CAD build for the part. Positions are in the model's coordinates, mm. Face numbers are marked on the shaded views. A direction names the side the tool comes from. Coordinates: 2 decimals unless noted, no trailing zeros. Write each loop counter-clockwise with the first axis right and the second up, starting at its lowest first coordinate (ties: lowest second). Pieces come first, ordered by that corner, then holes. Notation, with made-up numbers: (46.25, 82.5) -> (51.25, 82.5) arc R26 cw to (51.25, 113.5) -> close; hole circle Ø10 at (81.25, -1). An arc over 180 degrees is marked (long way). Answer as CSV lines item,"result".
```python
from build123d import *

# Parameters (mm, degrees)
EXTRUSION1_DEPTH = 35
ESQUISSE2_R      = 2
EXTRUSION2_DEPTH = 17
ESQUISSE4_R      = 1.5
ESQUISSE4_R_2    = 2.5
ESQUISSE4_W      = 17.5
ESQUISSE4_H      = 20
EXTRUSION3_DEPTH = 17


with BuildPart() as part:
    # Esquisse1 → Extrusion1 (new body)
    with BuildSketch(Plane.XY):
        Polygon((-13.454581117, 9.773157895), (-13.454581117, -10.226842105), (5.545418883, -10.226842105), (5.545418883, -8.726842105), (-11.954581117, -8.726842105), (-11.954581117, 9.773157895), align=None)
    extrude(amount=EXTRUSION1_DEPTH)

    # Esquisse2 → Extrusion2 (cut)
    with BuildSketch(Plane(origin=(-11.954581117, 0, 0), x_dir=(0, 0, -1), z_dir=(1, 0, 0))):
        with Locations(Location((-24.5, 6.273157895, 0), (0, 0, 90))):
            Circle(ESQUISSE2_R)
    extrude(amount=-EXTRUSION2_DEPTH, mode=Mode.SUBTRACT)

    # Esquisse4 → Extrusion3 (cut)
    with BuildSketch(Plane(origin=(0, -8.726842105, 0), x_dir=(-1, 0, 0), z_dir=(0, 1, 0))):
        with Locations((3.454581117, 10)):
            Circle(ESQUISSE4_R)
        with Locations((-5.545418883, 11.5)):
            Circle(ESQUISSE4_R_2)
        with Locations((3.204581117, 25)):
            Rectangle(ESQUISSE4_W, ESQUISSE4_H)
    extrude(amount=-EXTRUSION3_DEPTH, mode=Mode.SUBTRACT)


solid = part.part
```
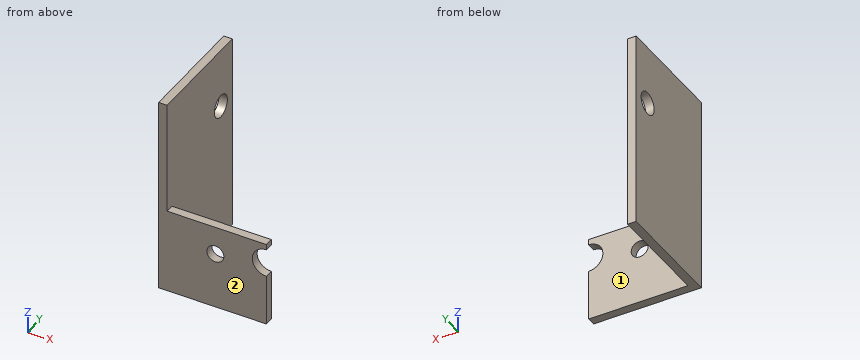
Item 1: Saw through at C-C on y = -0.75. Give the cut face in (x, z).
Answer below:
outline,"(-13.45, 0) -> (-11.95, 0) -> (-11.95, 35) -> (-13.45, 35) -> close"
Item 2: 3-axis set-ups, long thin cutter, end or side, ignore diameter. For the marked faces 1 and 2: which of +Z, -Z, +X, -X, +Y, -Y reach the whole face in a straight line?
Answer below:
face 1,"+Z, -Z, +X, +Y"
face 2,"+Z, -Z, +X, -X, -Y"
Item 3: Wall check: line 1 (X direction, y = -6, z = 4); line 2 (Y direction, x = -8, z = 7). Give the ranges that are in metal, low to high. Write a range as from..to.
Answer below:
line 1,"x = -13.45..-11.95"
line 2,"y = -10.23..-8.73"
Item 4: Saw through at B-B on x = -5.5. Give the cut face in (y, z), and give its area (3 significant figures).
Answer below:
outline,"(-10.23, 0) -> (-8.73, 0) -> (-8.73, 15) -> (-10.23, 15) -> close"
area,"22.5 mm2"
Item 5: Saw through at D-D on z = 2. Give the cut face in (x, y), and give its area (4 significant figures).
Answer below:
outline,"(-13.45, -10.23) -> (5.55, -10.23) -> (5.55, -8.73) -> (-11.95, -8.73) -> (-11.95, 9.77) -> (-13.45, 9.77) -> close"
area,"56.25 mm2"
Item 6: Flat gauge pins, fed straight in: pin 1 (4.5 mm diameter, centred on y = 6.27, z = 24.5, fed in from -X); pin 2 (4 mm diameter, centred on x = -3.45, z = 10, fed in from +Y); pin 3 (0.8 mm diameter, centred on x = -0.5, y = -10, fed in from +Z); pin 4 (12 mm diameter, centred on y = 5, z = 29.5, fed in from +X). Where does each tip first touch, or does it go through?
Answer below:
pin 1,"stops at x = -13.45"
pin 2,"stops at y = -8.73"
pin 3,"stops at z = 15"
pin 4,"stops at x = -11.95"
Item 7: Saw through at A-A on z = 24.5. Give the cut face in (x, y), and give its area (3 significant figures).
Answer below:
outline,"(-13.45, -10.23) -> (-11.95, -10.23) -> (-11.95, 4.27) -> (-13.45, 4.27) -> close; (-13.45, 8.27) -> (-11.95, 8.27) -> (-11.95, 9.77) -> (-13.45, 9.77) -> close"
area,"24.0 mm2"
